Part model, mm, in its own coordinate system. Face numbers are marked on the shaded views. A direction names the side the tool comes from. Round coordinates to 2 decimals unless told otherwise and drop trailing zeros. Loops run counter-clockwise (first coordinate to the right, second up) from the corner with the lowest first, then second, coordinate; pieces in that order, holes last. Notation, with made-up numbers: M 76,0 L 110,0 A9 ccw 110,16 Z; hole C 75,19.25 d10. An arc over 180 degrees is marked long. Write each question's results on one line, items separated by ' | '.
Autodesk Inventor part; units mm, degrees
ref_plane "Plan YZ" through (0, 0, 0) normal (1, 0, 0) x (0, 1, 0)
ref_plane "Plan XZ" through (0, 0, 0) normal (0, 1, 0) x (-1, 0, 0)
ref_plane "Plan XY" through (0, 0, 0) normal (0, 0, 1) x (1, 0, 0)
sketch "Esquisse1" plane through (0, 0, 0) normal (0, 0, 1) x (1, 0, 0)
  circle A0 centre (0, 0) radius 22
  line L0 (12.5, -6.7) -> (12.5, -8.4)
  line L1 (12.5, -8.4) -> (-12.5, -8.4)
  line L2 (-12.5, -8.4) -> (-12.5, -6.7)
  line L3 (-11, -6.7) -> (-11, 7.3)
  line L4 (11, -6.7) -> (11, 7.3)
  line L5 (-12.5, -6.7) -> (-11, -6.7)
  line L6 (12.5, -6.7) -> (11, -6.7)
  line L7 (-11, 7.3) -> (11, 7.3)
  line L8 (-20, 7) -> (-16, 7)
  line L9 (-16, 7) -> (-16, 4)
  line L10 (-16, 4) -> (-20, 4)
  line L11 (-20, 4) -> (-20, 7)
  line L12 (20, 7) -> (16, 7)
  line L13 (16, 7) -> (16, 4)
  line L14 (16, 4) -> (20, 4)
  line L15 (20, 4) -> (20, 7)
  line L16 (-30.8, 0) -> (30.8, 0) construction
  line L17 (0, -30.8) -> (0, 30.8) construction
  dimension "d0" = 44
  dimension "d17" = 1.5
  dimension "d23" = 3
  dimension "d24" = 4
  dimension "d25" = 32
  dimension "d38" = 4
  dimension "d43" = 1.7
  dimension "d44" = 14
  dimension "d47" = 25
  dimension "d57" = 6.7
extrude "Extrusion4" add sketch "Esquisse1" along normal blind 3
sketch "Esquisse7" plane through (0, 0, 3) normal (0, 0, 1) x (1, 0, 0)
  circle A0 centre (0, 0) radius 18.5 construction
  point P0 (-12.5, 13.6382)
  point P1 (12.5, 13.6382)
  point P2 (-10, -15.5644)
  point P3 (10, -15.5644)
  dimension "d58" = 37
  dimension "d59" = 25
  dimension "d60" = 20
hole "Perçage2" at (-12.5, 13.6382, 3) at (12.5, 13.6382, 3) at (-10, -15.5644, 3) at (10, -15.5644, 3) direction (0, 0, -1) diameter 3.4 end through all
properties part number "S1702_couverclereplat" material "Plastique PMMA"
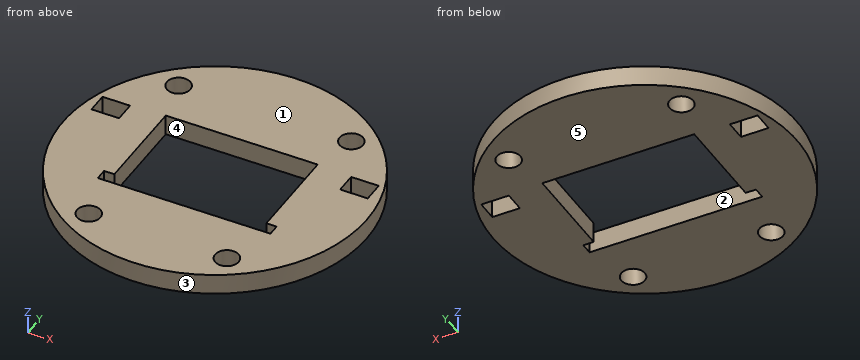
Item 1: Band-saw the part on A-A on z = 2.1. Give the cut face in (x, y).
Filled sheet:
outline: C 0,0 d44; hole M -20,4 L -16,4 L -16,7 L -20,7 Z; hole C -12.5,13.64 d3.4; hole M -12.5,-8.4 L 12.5,-8.4 L 12.5,-6.7 L 11,-6.7 L 11,7.3 L -11,7.3 L -11,-6.7 L -12.5,-6.7 Z; hole C -10,-15.56 d3.4; hole C 10,-15.56 d3.4; hole C 12.5,13.64 d3.4; hole M 16,4 L 20,4 L 20,7 L 16,7 Z
Item 2: Drop flat-ended pins along their axis: P1, Ø1.2, axis at x = -11.5, z = 1, coming from the -Y side; P2, Ø0.9, axis at y = 2.5, z = 1.5, coming from the -X side; P3, Ø1.4, axis at y = -7.5, z = 1.5, coming from the -X side. Give the stop position or say it passes through.
Filled sheet:
P1: y = -19.11 | P2: x = -21.9 | P3: x = -20.92
Item 3: Wall check: L1, parallel to Y at x = 10, z = 1.3; L2, parallel to Y at x = 9, z = 2.95; L3, parallel to Y at x = 5, z = 2.85. Give the ranges that are in metal, low to high.
Filled sheet:
L1: -19.6 to -17.26, -13.86 to -8.4, 7.3 to 19.6 | L2: -20.07 to -16.94, -14.19 to -8.4, 7.3 to 20.07 | L3: -21.42 to -8.4, 7.3 to 21.42
Item 4: Band-saw the part on B-B on x = 0. Give the cut face in (y, z).
Filled sheet:
outline: M -22,0 L -8.4,0 L -8.4,3 L -22,3 Z; M 7.3,0 L 22,0 L 22,3 L 7.3,3 Z
Item 5: Which spindle directions (+Z, -Z, +X, -X, +Y, -Y) get a long thin tool onto all of the face, cutting with end or side? Do the marked faces 1 and 2. Say none if no direction does.
Filled sheet:
face 1: +Z, +X, -X, +Y, -Y | face 2: +Z, -Z
Item 6: Band-saw the part on C-C on y = -3. Give the cut face in (x, z), and give its area (3 significant figures).
Filled sheet:
outline: M -21.79,0 L -11,0 L -11,3 L -21.79,3 Z; M 11,0 L 21.79,0 L 21.79,3 L 11,3 Z | area: 64.8 mm^2
Item 7: Band-saw the part on D-D on x = 10. Give the cut face in (y, z).
Filled sheet:
outline: M -19.6,0 L -17.26,0 L -17.26,3 L -19.6,3 Z; M -13.86,0 L -8.4,0 L -8.4,3 L -13.86,3 Z; M 7.3,0 L 19.6,0 L 19.6,3 L 7.3,3 Z
Item 8: Two-plate mould, pull along X, no slides. Class the marked faces 3, 4 and 5: +X half, -X half, draft (parallel to the pull), parting line (faces both ways), or undercut.
Filled sheet:
face 3: parting line | face 4: undercut | face 5: draft
